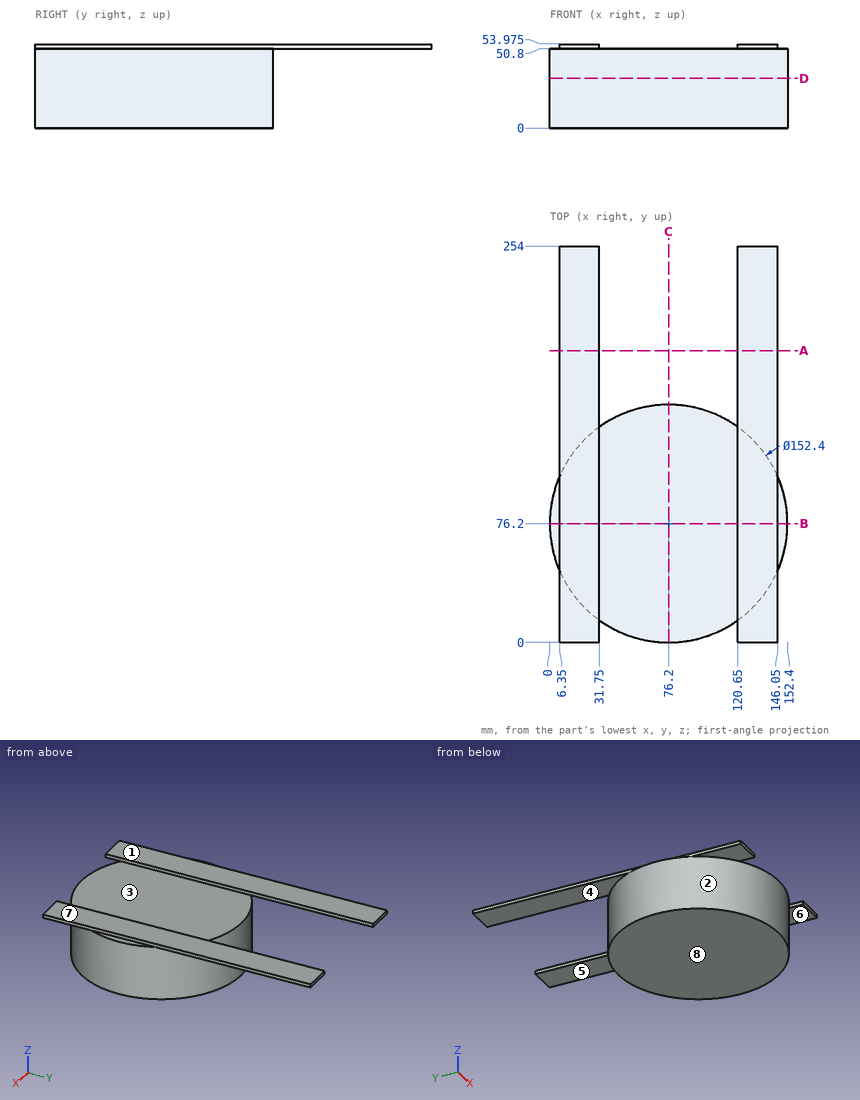
Drawing for the job (mm, zero at the part's lowest x, y, z). A direction names the side the tool comes from. Round coordinates to 2 decimals unless told otherwise and drop trailing zeros. Loops run counter-clockwise (first coordinate to the right, second up) from the corner with the lowest first, then second, coordinate; pieces in that order, holes last. Notation, with made-up numbers: (51.5, 0) -> (101.5, 0) arc R22 ccw to (101.5, 24) -> close; hole circle Ø8 at (-38.75, 37). An arc over 180 degrees is marked (long way). Use one line per item in the form item = value. Start each with the question number.
Item 1: Drill centre lines: line 1 along Z through (x, y) = (52.5, 105); line 2 along Z through (x, y) = (125, 142) (3 decimals); line 3 along Y through (x, z) = (77.5, 39.5). Where is each one in solid material? Low to high.
Item 2: Tool access for the marked faces 4, 5, 6, 7 and 8: list every direction of +Z, -Z, +X, -X, +Y, -Y with a clear straight run to the whole face (end or side of a thin tool).
Item 3: Band-saw the part on D-D (z = 32). List the corners of the cut face in (x, y), plus the area to 3 significant figures.
Item 4: Band-saw the part on B-B (y = 76.2). List the corners of the cut face in (x, z) (3 decimals), plus the area to 3 significant figures.
Item 5: Drop flat-ended pins along their axis: pin 1 Ø2.5 at (y, z) = (177.5, 52.5) entering from +X; pin 2 Ø4 at (x, z) = (93.5, 35.5) entering from +Y; pin 3 Ø8 at (y, z) = (94, 11) entering from +X. Give the stop position or say it passes through.
Item 6: Band-saw the part on C-C (x = 76.2). List the corners of the cut face in (y, z), plus the area to 3 significant figures.
Item 7: Two-plate mould, pull along X, no slides. Class the marked faces 1, 2 and 3: released by +X, released by -X, zero draft, split by the parting line, or undercut.
Item 8: Band-saw the part on A-A (y = 187). List the corners of the cut face in (x, z) (3 decimals).
Data:
q1.line_1 = 0 to 50.8
q1.line_2 = 50.8 to 53.975
q1.line_3 = 0.01 to 152.39
q2.face_4 = -Z, -X, +Y
q2.face_5 = -Z, +X, +Y
q2.face_6 = -Z, +X, -Y
q2.face_7 = +Z, +X, -X, +Y, -Y
q2.face_8 = -Z, +X, -X, +Y, -Y
q3.outline = circle Ø152.4 at (76.2, 76.2)
q3.area = 18,200 mm^2
q4.outline = (0, 0) -> (152.4, 0) -> (152.4, 50.8) -> (146.05, 50.8) -> (146.05, 53.975) -> (120.65, 53.975) -> (120.65, 50.8) -> (31.75, 50.8) -> (31.75, 53.975) -> (6.35, 53.975) -> (6.35, 50.8) -> (0, 50.8) -> close
q4.area = 7,900 mm^2
q5.pin_1 = 146.05
q5.pin_2 = 150.85
q5.pin_3 = 151.14
q6.outline = (0, 0) -> (152.4, 0) -> (152.4, 50.8) -> (0, 50.8) -> close
q6.area = 7,740 mm^2
q7.face_1 = zero draft
q7.face_2 = split by the parting line
q7.face_3 = undercut
q8.outline = (6.35, 50.8) -> (31.75, 50.8) -> (31.75, 53.975) -> (6.35, 53.975) -> close; (120.65, 50.8) -> (146.05, 50.8) -> (146.05, 53.975) -> (120.65, 53.975) -> close
